```python
from build123d import *

# Parameters (mm, degrees)
BOSS_EXTRUDE1_DEPTH = 3
SKETCH2_R           = 1.35
CUT_EXTRUDE1_DEPTH  = 77.380625816


with BuildPart() as part:
    # Sketch1 → Boss-Extrude1 (new body)
    with BuildSketch(Plane.XY):
        with BuildLine():
            Line((3, 0), (17.95, -0.01))
            Line((17.95, -0.01), (17.95, 5.2))
            Line((17.95, 5.2), (22.025, 5.2))
            Line((22.025, 5.2), (22.025, -0.01))
            Line((22.025, -0.01), (37, 0))
            ThreePointArc((37, 0), (39.121320344, 0.878679656), (40, 3))
            Line((40, 3), (40, 62))
            ThreePointArc((40, 62), (39.121320344, 64.121320344), (37, 65))
            Line((37, 65), (22.05, 65))
            Line((22.05, 65), (22.05, 59.775))
            Line((22.05, 59.775), (17.975, 59.775))
            Line((17.975, 59.775), (17.975, 65))
            Line((17.975, 65), (3, 65))
            ThreePointArc((3, 65), (0.878679656, 64.121320344), (0, 62))
            Line((0, 62), (0, 3))
            ThreePointArc((0, 3), (0.878679656, 0.878679656), (3, 0))
        make_face()
    extrude(amount=BOSS_EXTRUDE1_DEPTH)

    # Sketch2 → Cut-Extrude1 (cut, through all)
    with BuildSketch(Plane.XY.offset(3)):
        with Locations((3, 3)):
            Circle(SKETCH2_R)
        with Locations((37, 3)):
            Circle(SKETCH2_R)
        with Locations((37, 62)):
            Circle(SKETCH2_R)
        with Locations((3, 62)):
            Circle(SKETCH2_R)
    extrude(amount=-CUT_EXTRUDE1_DEPTH, mode=Mode.SUBTRACT)


solid = part.part
```
Geometry check sheet. Reference: the model listing, model coordinates, mm. A direction names the side the tool comes from. Round coordinates to 2 decimals unless told otherwise and drop trailing zeros. Order: outer loops, then holes, each group sorted by start corner. A loop starts at its lowest first (then second) coordinate and runs counter-clockwise, first axis right, second up. Notation, with made-up numbers: (0.25, 45) -> (41.25, 45) arc R21 cw to (41.25, 73) -> close; hole circle Ø10 at (58, 61). An arc over 180 degrees is marked (long way). Return JSON: item names as keys, results as strings. Group by question number.
Q1. Material ranges on probe 1 along Y at (x, z) = (3, 1.55); probe 2 along Y at (x, z) = (24, 2.4), recorded low to high. Write a range as from..to.
Q2. Section check A-A, the plane z = 2.05. Record the boundary of the cut face in (x, y) (3 decimals), plus the area to 3 significant figures.
Q3. Release check for a two-part mould opening along Y. For faces 1 (the flat face through (20, 59.775, 1)), 2 (the flat face through (22.025, 3, 1)), 3 (the cylindrical face through (2.71, 60.68, 1.52)), 4 (the cylindrical face through (3.62, 1.8, 1.52)) record: released by +Y, released by -Y, zero draft, split by the parting line, or undercut.
Q4. Tool access check on faces 5 (the cylindrical face through (36.71, 1.68, 1.52)), 6 (the flat face through (20, 5.2, 1)), 7 (the flat face through (22.05, 62, 1)). Record the directions out of +Z, -Z, +X, -X, +Y, -Y that give a thin tool (end or side, any length) a straight path to the whole face; none if there is none.
Q5. Gauge pin test, flat ends, axial feed: pin 1 (2 mm diameter, centred on x = 24, y = 39, fed in from -Z); pin 2 (1.5 mm diameter, centred on x = 6, z = 0.5, fed in from -Y); pin 3 (0.9 mm diameter, centred on x = 19, z = 1.5, fed in from +Y) (3 decimals); pin 4 (1.6 mm diameter, centred on x = 37, y = 62, fed in from +Z). Record the tip position at first contact, or that the pin passes through.
Numbers:
{
 "1": {"probe 1": "0..1.65, 4.35..60.65, 63.35..65", "probe 2": "-0.01..65"},
 "2": {"outline": "(0, 3) arc R3 ccw to (3, 0) -> (17.95, -0.01) -> (17.95, 5.2) -> (22.025, 5.2) -> (22.025, -0.01) -> (37, 0) arc R3 ccw to (40, 3) -> (40, 62) arc R3 ccw to (37, 65) -> (22.05, 65) -> (22.05, 59.775) -> (17.975, 59.775) -> (17.975, 65) -> (3, 65) arc R3 ccw to (0, 62) -> close; hole circle Ø2.7 at (3, 3); hole circle Ø2.7 at (3, 62); hole circle Ø2.7 at (37, 3); hole circle Ø2.7 at (37, 62)", "area": "2,530 mm^2"},
 "3": {"face 1": "released by +Y", "face 2": "zero draft", "face 3": "undercut", "face 4": "undercut"},
 "4": {"face 5": "+Z, -Z", "face 6": "+Z, -Z, -Y", "face 7": "+Z, -Z, +Y"},
 "5": {"pin 1": "z = 0", "pin 2": "y = 0", "pin 3": "y = 59.775", "pin 4": "through"}
}
